from build123d import *

# Parameters (mm, degrees)
SKETCH_1_W                      = 440
SKETCH_1_H                      = 440
SKETCH_1_W_2                    = 430
SKETCH_1_H_2                    = 430
EXTRUDE_1_DEPTH                 = 360
SKETCH_2_W                      = 440
SKETCH_2_H                      = 440
EXTRUDE_2_DEPTH                 = 5
SKETCH_3_W                      = 440
SKETCH_3_H                      = 440
SKETCH_3_W_2                    = 410
SKETCH_3_H_2                    = 410
EXTRUDE_3_DEPTH                 = 5
CUT_EXTRUDE_1_REACH             = 434.204
CUT_EXTRUDE_1_DIRECTION_2_REACH = 434.204


with BuildPart() as part:
    # Эскиз1 → Бобышка-Вытянуть1 (new body)
    with BuildSketch(Plane(origin=(0, -60, 0), x_dir=(1, 0, 0), z_dir=(0, 1, 0))):
        Rectangle(SKETCH_1_W, SKETCH_1_H)
        Rectangle(SKETCH_1_W_2, SKETCH_1_H_2, mode=Mode.SUBTRACT)
    extrude(amount=EXTRUDE_1_DEPTH)

    # Эскиз2 → Бобышка-Вытянуть2 (add)
    with BuildSketch(Plane(origin=(0, -60, 0), x_dir=(1, 0, 0), z_dir=(0, 1, 0))):
        Rectangle(SKETCH_2_W, SKETCH_2_H)
    extrude(amount=EXTRUDE_2_DEPTH)

    # Эскиз3 → Бобышка-Вытянуть3 (add)
    with BuildSketch(Plane(origin=(0, 300, 0), x_dir=(1, 0, 0), z_dir=(0, 1, 0))):
        Rectangle(SKETCH_3_W, SKETCH_3_H)
        Rectangle(SKETCH_3_W_2, SKETCH_3_H_2, mode=Mode.SUBTRACT)
    extrude(amount=-EXTRUDE_3_DEPTH)

    # Вырез-Вытянуть1: up to this face of the body (flat: up to its plane)
    cut_extrude_1_end = Plane(part.part.faces().sort_by_distance((0, 297.5, -205))[0])
    # Эскиз4 → Вырез-Вытянуть1 (cut, up to the picked face)
    with BuildSketch(Plane.XY, mode=Mode.PRIVATE) as cut_extrude_1_sk1:
        with BuildLine():
            Line((-205, 295), (-205, 300))
            Line((-205, 300), (-207.5, 300))
            Line((-207.5, 300), (-207.5, 297.5))
            ThreePointArc((-207.5, 297.5), (-206.767766953, 295.732233047), (-205, 295))
        make_face()
    cut_extrude_1_tool1 = split(extrude(cut_extrude_1_sk1.sketch, amount=-CUT_EXTRUDE_1_REACH, mode=Mode.PRIVATE), bisect_by=cut_extrude_1_end, keep=Keep.BOTH, mode=Mode.PRIVATE)
    add(cut_extrude_1_tool1.solids().sort_by(Axis((-206.166873, 297.733375, 0), (0, 0, -1)))[0], mode=Mode.SUBTRACT)

    # Вырез-Вытянуть1 direction 2: up to this face of the body (flat: up to its plane)
    cut_extrude_1_direction_2_end = Plane(part.part.faces().sort_by_distance((0, 297.5, 205))[0])
    # Эскиз4 → Вырез-Вытянуть1 direction 2 (cut, up to the picked face)
    with BuildSketch(Plane.XY, mode=Mode.PRIVATE) as cut_extrude_1_direction_2_sk1:
        with BuildLine():
            Line((-205, 295), (-205, 300))
            Line((-205, 300), (-207.5, 300))
            Line((-207.5, 300), (-207.5, 297.5))
            ThreePointArc((-207.5, 297.5), (-206.767766953, 295.732233047), (-205, 295))
        make_face()
    cut_extrude_1_direction_2_tool1 = split(extrude(cut_extrude_1_direction_2_sk1.sketch, amount=CUT_EXTRUDE_1_DIRECTION_2_REACH, mode=Mode.PRIVATE), bisect_by=cut_extrude_1_direction_2_end, keep=Keep.BOTH, mode=Mode.PRIVATE)
    add(cut_extrude_1_direction_2_tool1.solids().sort_by(Axis((-206.166873, 297.733375, 0), (0, 0, 1)))[0], mode=Mode.SUBTRACT)


solid = part.part
Verification items for the finished model (mm, model axes). A direction names the side the tool comes from. Give positions to 0.01 mm unless a question says otherwise; leave off trailing zeros. Write each loop counter-clockwise with the first axis right and the second up, starting at its lowest first coordinate (ties: lowest second). Pieces come first, ordered by that corner, then holes.
(1) Material ranges on line 1 (X direction, y = 39.5, z = 95); line 2 (Y direction, x = 23, z = -115.5), recorded low to high.
(2) Access from +Z, -Z, +X, -X, +Y, -Y to the whole of each face (thin tool, end or side, straight path). Record for faces 1 (the face through (-3, 117, -220)), 2 (the face through (-215, 118, 3)).
(3) Cross-section at A-A (y = 237.5). Enter the section's corners in (x, z), plus the area to 3 significant figures.
(4) Cross-section at B-B (x = -77.5). Enter the section's corners in (y, z), plus the area to 3 significant figures.
(5) Cross-section at C-C (z = 109). Enter the section's corners in (x, y).
(6) Gauge pin test, flat end, axial feed: pin 1 (3 mm diameter, centred on x = -90.5, z = 153.5, fed in from +Y). Record the tip position at first contact, or that the pin passes through.
(7) Mould release check, pull along X, two halves, no side actions. Record for faces 3 (the face through (215, 118, 3)), 4 (the face through (-220, 117, 3)), 5 (the face through (-3, 117, 220)): +X half, -X half, draft (parallel to the pull), parting line (faces both ways), or undercut.
Worked out:
1. line 1: x = -220 to -215, 215 to 220
1. line 2: y = -60 to -55
2. face 1: -Z, +X, -X, +Y, -Y
2. face 2: none
3. outline: (-220, -220) - (220, -220) - (220, 220) - (-220, 220) - close; hole (-215, -215) - (215, -215) - (215, 215) - (-215, 215) - close
3. area: 8,700 mm2
4. outline: (-60, -220) - (300, -220) - (300, -205) - (295, -205) - (295, -215) - (-55, -215) - (-55, 215) - (295, 215) - (295, 205) - (300, 205) - (300, 220) - (-60, 220) - close
4. area: 5,850 mm2
5. outline: (-220, -60) - (220, -60) - (220, 300) - (205, 300) - (205, 295) - (215, 295) - (215, -55) - (-215, -55) - (-215, 295) - (-205, 295) arc R2.5 cw to (-207.5, 297.5) - (-207.5, 300) - (-220, 300) - close
6. pin 1: stops at y = -55
7. face 3: undercut
7. face 4: -X half
7. face 5: draft
